Design review of the part built by this model. Coordinates are the model's own, in mm. A direction names the side the tool comes from. Coordinates: 2 decimals unless noted, no trailing zeros. Loops run counter-clockwise (first coordinate to the right, second up) from the corner with the lowest first, then second, coordinate; pieces in that order, holes last. Notation, with made-up numbers: (18.25, 0.25) - (36.25, 0.25) arc R31 ccw to (36.25, 28.25) - close; hole circle Ø6 at (39.5, 89). An arc over 180 degrees is marked (long way). Answer in a Markdown table with one row per item. Add a question column.
(1) The part is to be moulded in two halves that separate along Y. For faces 1 (the face through (0, 6, 2)), 2 (the face through (0, -6, -3)), 3 (the face through (-0.867, -3.905, 1.972)), 4 (the face through (3, 3, 0)), say which applies: released by +Y, released by -Y, zero draft, split by the parting line, or undercut.
(2) We need section D-D, the plane y = 3.75. Write out the cut boundary in (x, z), plus the area to 3 significant figures.
(3) To check wall thickness, follow L1, parallel to Y at x = 0, z = 2.45; L2, parallel to Z at x = -3, y = 4.5; L3, parallel to Y at x = -1, z = -9. State the ranges of each line that lie inside material, in increasing order. Write a range as [from, to].
(4) We need section B-B, the plane y = -2.5. Write out the cut boundary in (x, z).
(5) For faces 5 (the face through (1.42, -3.92, 4)), 6 (the face through (0, -4.5, -5)), list the 3-axis set-ups (+Z, -Z, +X, -X, +Y, -Y) from which the entire face can be reached by the end or side of a thin tool; tool diameter is ignored.
(6) We need section A-A, the plane x = 0. Write out the cut boundary in (y, z), plus the area to 3 significant figures.
(7) We need section C-C, the plane x = 3. Write out the cut boundary in (y, z), plus the area to 3 significant figures.
(8) Clearance check with flat-ended pins moving along their axes: pin 1 (2 mm diameter, centred on x = 1, z = -5.5, fed in from +Y); pin 2 (2 mm diameter, centred on x = 2.5, y = -2.5, fed in from +Z); pin 3 (3 mm diameter, centred on x = 3, y = -2.5, fed in from -Z). State where each tip first meets the part, or that it passes through.
from build123d import *

# Parameters (mm, degrees)
SKETCH1_R           = 4
BOSS_EXTRUDE1_DEPTH = 4
SKETCH2_W           = 12
SKETCH2_H           = 1.5
BOSS_EXTRUDE2_DEPTH = 10


with BuildPart() as part:
    # Sketch1 → Boss-Extrude1 (new body)
    with BuildSketch(Plane.XY):
        with BuildLine():
            Line((0, -6), (-6, -6))
            Line((-6, -6), (-6, 0))
            ThreePointArc((-6, 0), (0, 6), (6, 0))
            Line((6, 0), (6, -6))
            Line((6, -6), (0, -6))
        make_face()
        Circle(SKETCH1_R, mode=Mode.SUBTRACT)
    extrude(amount=BOSS_EXTRUDE1_DEPTH)

    # Sketch2 → Boss-Extrude2 (add)
    with BuildSketch(Plane(origin=(0, 0, 0), x_dir=(-1, 0, 0), z_dir=(0, 0, -1))):
        with Locations((0, -5.25)):
            Rectangle(SKETCH2_W, SKETCH2_H)
    extrude(amount=BOSS_EXTRUDE2_DEPTH)


solid = part.part
Responses:
| question | item | result |
|---|---|---|
| 1 | face 1 | released by +Y |
| 1 | face 2 | released by -Y |
| 1 | face 3 | undercut |
| 1 | face 4 | zero draft |
| 2 | outline | (-4.68, 0) - (-1.39, 0) - (-1.39, 4) - (-4.68, 4) - close; (1.39, 0) - (4.68, 0) - (4.68, 4) - (1.39, 4) - close |
| 2 | area | 26.3 mm2 |
| 3 | L1 | y = [-6, -4], [4, 6] |
| 3 | L2 | z = [0, 4] |
| 3 | L3 | y = [-6, -4.5] |
| 4 | outline | (-6, 0) - (-3.12, 0) - (-3.12, 4) - (-6, 4) - close; (3.12, 0) - (6, 0) - (6, 4) - (3.12, 4) - close |
| 5 | face 5 | +Z, +X, -X, +Y, -Y |
| 5 | face 6 | -Z, +X, -X, +Y |
| 6 | outline | (-6, -10) - (-4.5, -10) - (-4.5, 0) - (-4, 0) - (-4, 4) - (-6, 4) - close; (4, 0) - (6, 0) - (6, 4) - (4, 4) - close |
| 6 | area | 31.0 mm2 |
| 7 | outline | (-6, -10) - (-4.5, -10) - (-4.5, 0) - (-2.65, 0) - (-2.65, 4) - (-6, 4) - close; (2.65, 0) - (5.2, 0) - (5.2, 4) - (2.65, 4) - close |
| 7 | area | 38.6 mm2 |
| 8 | pin 1 | stops at y = -4.5 |
| 8 | pin 2 | stops at z = 4 |
| 8 | pin 3 | stops at z = 0 |
